Autodesk Inventor part; units mm, degrees
ref_plane "YZ Plane" through (0, 0, 0) normal (1, 0, 0) x (0, 1, 0)
ref_plane "XZ Plane" through (0, 0, 0) normal (0, 1, 0) x (-1, 0, 0)
ref_plane "XY Plane" through (0, 0, 0) normal (0, 0, 1) x (1, 0, 0)
sketch "スケッチ1" plane through (0, 0, 0) normal (0, 1, 0) x (-1, 0, 0)
  line L0 (105, 70) -> (-105, 70)
  line L1 (-105, 70) -> (-105, -70)
  line L2 (-105, -70) -> (105, -70)
  line L3 (105, -70) -> (105, 70)
  line L4 (105, 70) -> (-105, -70) construction
  line L5 (-105, 70) -> (105, -70) construction
  circle A0 centre (0, -30) radius 77
  circle A1 centre (0, -30) radius 9
  line L6 (-105, -30) -> (105, -30)
  circle A2 centre (48, -30) radius 12.5
  circle A3 centre (-39, -30) radius 6
  circle A4 centre (48, -30) radius 17.5
  circle A5 centre (-39, -30) radius 9
  circle A6 centre (0, -30) radius 86.5
  line L7 (66.5, -30) -> (66.5, -62.5)
  line L8 (66.5, -30) -> (66.5, 2.5)
  line L9 (-26, -30) -> (-26, -47.5)
  line L10 (-26, -30) -> (-26, -12.5)
  circle A7 centre (65.5, -30) radius 2
  circle A8 centre (48, -12.5) radius 2
  circle A9 centre (30.5, -30) radius 2
  circle A10 centre (48, -47.5) radius 2
  circle A11 centre (-39, -39) radius 1.6
  circle A12 centre (-39, -21) radius 1.6
  circle A13 centre (-26, -47.5) radius 2
  circle A14 centre (-26, -12.5) radius 2
  circle A15 centre (66.5, -62.5) radius 2
  circle A16 centre (66.5, 2.5) radius 2
  circle A17 centre (86.5, -30) radius 2
  circle A18 centre (43.25, 44.9112) radius 2
  circle A19 centre (-43.25, 44.9112) radius 2
  circle A20 centre (-86.5, -30) radius 2
  line L11 (76.6958, -70) -> (0, -55)
  line L12 (0, -55) -> (-76.6958, -70)
  line L13 (100, -70) -> (100, 70)
  line L14 (-100, -70) -> (-100, 70)
  point P0 (0, 0)
  point P1 (-43.25, -104.9112)
  point P2 (43.25, -104.9112)
  point P3 (100, -65)
  point P4 (100, 0)
  point P5 (100, 65)
  point P6 (-100, -65)
  point P7 (-100, 0)
  point P8 (-100, 65)
  dimension "d9" = 35
  dimension "d0" = 210
  dimension "d1" = 140
  dimension "d2" = 100
  dimension "d3" = 154
  dimension "d4" = 18
  dimension "d5" = 48
  dimension "d6" = 39
  dimension "d7" = 25
  dimension "d8" = 12
  dimension "d10" = 18
  dimension "d11" = 173
  dimension "d14" = 360
  dimension "d16" = 18.5
  dimension "d17" = 32.5
  dimension "d18" = 32.5
  dimension "d20" = 13
  dimension "d21" = 17.5
  dimension "d22" = 17.5
  dimension "d25" = 360
  dimension "d27" = 4
  dimension "d28" = 4
  dimension "d29" = 4
  dimension "d30" = 4
  dimension "d31" = 3.2
  dimension "d32" = 3.2
  dimension "d33" = 4
  dimension "d34" = 4
  dimension "d35" = 4
  dimension "d36" = 4
  dimension "d37" = 4
  dimension "d38" = 4
  dimension "d39" = 4
  dimension "d40" = 4
  dimension "d41" = 15
  dimension "d45" = 5
  dimension "d46" = 5
  dimension "d47" = 5
  dimension "d48" = 5
  dimension "d49" = 5
  dimension "d50" = 5
  dimension "d51" = 5
  dimension "d52" = 5
extrude "押し出し1" add sketch "スケッチ1" along normal blind 3 contours L3 L6 L13 L0 | L13 L6 A17 A6 A18 A19 A20 L14 L0 | L3 L2 L13 L6 | L14 L6 L1 L0 | L13 L2 A6 A17 L6 | L14 L2 L1 L6 | L6 A20 A6 L2 L14 | A17 L6 A0 A20 A6 A19 A18 | A6 L11 A0 L6 A17 | A20 L6 A0 L12 A6 | L11 L12 A0 L6 A5 A11 A1 A9 A4 A10 A7 | L6 A7 A4 A8 A9 A1 A5 A12 A0 | A7 L7 L6 | L6 L8 A7 | A5 A12 L6 A3 | L6 A3 A5 A11 | L7 A7 A4 L6 | L6 A4 A7 L8 | A3 L6 | L6 A3 | A12 A5 | A5 A12 | A11 A5 | A5 A11 | A4 A7 L6 | L6 A7 A4 | A7 L6 A2 A9 A4 A8 | A4 A10 A9 L6 A2 A7 | A8 A4 | A4 A8 | A10 A4 | A4 A10 | A2 L6 | L6 A2 | A9 L6 A4 | A4 L6 A9 | A9 L6 A4 | A4 L6 A9
fillet "フィレット1" radius 4 7 edges at (-105, 1.5, 70) (-105, 1.5, -70) (-76.6958, 1.5, -70) (0, 1.5, -55) (76.6958, 1.5, -70) (105, 1.5, -70) (105, 1.5, 70)
hole "穴1" at (-100, 0, 65) at (-100, 0, 0) at (-100, 0, -65) at (100, 0, -65) at (100, 0, 0) at (100, 0, 65) direction (0, 1, 0) diameter 3.2 end through all
sketch "スケッチ3" plane through (0, 3, 0) normal (0, 1, 0) x (1, 0, 0)
  circle A0 centre (100, -65) radius 1.6
  circle A1 centre (100, 0) radius 1.6
  circle A2 centre (100, 65) radius 1.6
  circle A3 centre (-100, 65) radius 1.6
  circle A4 centre (-100, 0) radius 1.6
  circle A5 centre (-100, -65) radius 1.6
  arc A6 (101, -70) -> (105, -66) centre (101, -66) ccw
  line L0 (105, -66) -> (105, 66)
  arc A7 (105, 66) -> (101, 70) centre (101, 66) ccw
  line L1 (101, 70) -> (77.0833, 70)
  arc A8 (77.0833, 70) -> (76.3155, 69.9256) centre (77.0833, 66) ccw
  line L2 (76.3155, 69.9256) -> (0.7678, 55.1502)
  arc A9 (-0.7678, 55.1502) -> (0.7678, 55.1502) centre (0, 59.0758) ccw
  line L3 (-0.7678, 55.1502) -> (-76.3155, 69.9256)
  arc A10 (-76.3155, 69.9256) -> (-77.0833, 70) centre (-77.0833, 66) ccw
  line L4 (-77.0833, 70) -> (-101, 70)
  arc A11 (-101, 70) -> (-105, 66) centre (-101, 66) ccw
  line L5 (-105, 66) -> (-105, -66)
  arc A12 (-105, -66) -> (-101, -70) centre (-101, -66) ccw
  line L6 (-101, -70) -> (101, -70)
  circle A13 centre (43.25, -44.9112) radius 2
  circle A14 centre (-43.25, -44.9112) radius 2
  circle A15 centre (-86.5, 30) radius 2
  circle A16 centre (-66.5, 62.5) radius 2
  circle A17 centre (-66.5, -2.5) radius 2
  circle A18 centre (0, 30) radius 9
  circle A19 centre (26, 47.5) radius 2
  circle A20 centre (26, 12.5) radius 2
  circle A21 centre (86.5, 30) radius 2
  point P0 (0, 0)
properties part number "ローラー_板"
The listing builds one solid part. Answer for the finished solid, in the listing's coordinates (mm). A direction names the side the tool comes from. Round coordinates to 2 decimals unless told otherwise and drop trailing zeros. Loops run counter-clockwise (first coordinate to the right, second up) from the corner with the lowest first, then second, coordinate; pieces in that order, holes last.
1) A cutting plane is placed at B-B on x = -6. Determine the outline of the cut face in (y, z).
Outcome:
outline: (0, -56.17) - (3, -56.17) - (3, -36.71) - (0, -36.71) - close; (0, -23.29) - (3, -23.29) - (3, 70) - (0, 70) - close
2) For faces 1 (the face through (-103.797, 1.521, -68.859)), 2 (the face through (-39.07, 1.48, -62.64)), determine the directions among +Z, -Z, +X, -X, +Y, -Y from which every point of the face is accessible in a straight line to the end or side of a thin tool.
Outcome:
face 1: -Z, -X, +Y, -Y
face 2: -Z, +Y, -Y
3) Given P1, Ø6.5, axis at x = -66.5, z = -62.5, coming from the -Y side, flat-ended and moving along its own axis, determine where the tip first touches the part or whether it passes through.
Outcome:
P1: stops at y = 0
4) A cutting plane is placed at A-A on y = 0.7. Give the number of separate pieces and of enclosed holes in the cut face, plus the area to 3 significant figures.
Outcome:
separate pieces: 1
enclosed holes: 15
area: 27,800 mm2
5) Consider line 1 (Z direction, x = 100, y = 1.05); line 2 (X direction, y = 2.2, z = -30); line 3 (Z direction, x = -86.5, y = 1.9). Determine where each line is inside the solid, lowest interval first.
Outcome:
line 1: z = -70 to -66.6, -63.4 to -1.6, 1.6 to 63.4, 66.6 to 70
line 2: x = -105 to -88.5, -84.5 to -9, 9 to 84.5, 88.5 to 105
line 3: z = -70 to -32, -28 to 70
